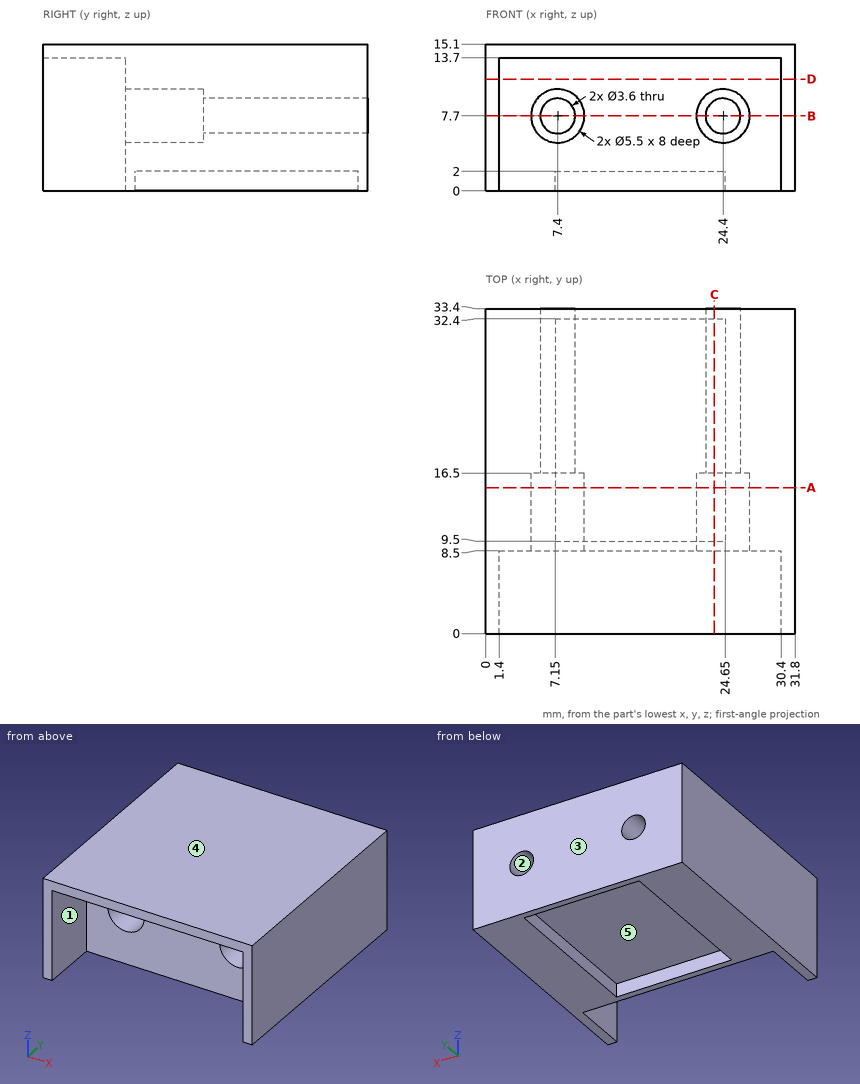
Geometry check sheet. Reference: drawing and pictorial views, mm from the part's lowest x, y, z. A direction names the side the tool comes from. Coordinates: 2 decimals unless noted, no trailing zeros. Order: outer loops, then holes, each group sorted by start corner. A loop starts at its lowest first (then second) coordinate and runs counter-clockwise, first axis right, second up. Notation, with made-up numbers: (41, -19.5) -> (78, -19.5) arc R19 ccw to (78, 2.5) -> close; hole circle Ø10 at (45, -16). An arc over 180 degrees is marked (long way). Use CSV: the item, a comma, the result in double quotes. Start each with the question number.
Q1. Section check C-C, the plane x = 23.5. Record the cut outline in (y, z), and give its area (3 significant figures).
Q2. Section check B-B, the plane z = 7.7. Record the cut outline in (x, y), and give its area (3 significant figures).
Q3. Section check D-D, the plane z = 11.5. Record the cut outline in (x, y), and give its area (3 significant figures).
Q4. Draft check along Y on the marked faces 3, 4 and 5. Enter one of: +Y half, -Y half, draft (parallel to the pull), parting line (faces both ways), or undercut.
Q5. Section check A-A, the plane y = 15. Record the cut outline in (x, z).
Q6. Thickness scan on line 1 along Z through (x, y) = (24.4, 11); line 2 along X through (y, z) = (4.5, 3.75); line 3 along Z through (x, y) = (24.4, 27.5). Record the ranges inside material, lowest first.
Q7. Depth check by flat-ended pin: P1, Ø4.5, axis at x = 23.5, z = 8, coming from the -Y side; P2, Ø4.5, axis at x = 7.4, z = 7.7, coming from the -Y side; P3, Ø2, axis at x = 24.4, z = 7.7, coming from the -Y side; P4, Ø5, axis at x = 13.5, y = 17.5, coming from the -Z side. Enter the tip coordinate at first touch or a pass-through.
Q8. Tool access check on the marked faces 1 and 2. Record the directions out of +Z, -Z, +X, -X, +Y, -Y that give a thin tool (end or side, any length) a straight path to the whole face; none if there is none.
Returned:
1,outline,"(0, 13.7) -> (8.5, 13.7) -> (8.5, 10.3) -> (16.5, 10.3) -> (16.5, 9.26) -> (33.4, 9.26) -> (33.4, 15.1) -> (0, 15.1) -> close; (8.5, 0) -> (9.5, 0) -> (9.5, 2) -> (32.4, 2) -> (32.4, 0) -> (33.4, 0) -> (33.4, 6.14) -> (16.5, 6.14) -> (16.5, 5.1) -> (8.5, 5.1) -> close"
1,area,"248 mm^2"
2,outline,"(0, 0) -> (1.4, 0) -> (1.4, 8.5) -> (4.65, 8.5) -> (4.65, 16.5) -> (5.6, 16.5) -> (5.6, 33.4) -> (0, 33.4) -> close; (9.2, 16.5) -> (10.15, 16.5) -> (10.15, 8.5) -> (21.65, 8.5) -> (21.65, 16.5) -> (22.6, 16.5) -> (22.6, 33.4) -> (9.2, 33.4) -> close; (26.2, 16.5) -> (27.15, 16.5) -> (27.15, 8.5) -> (30.4, 8.5) -> (30.4, 0) -> (31.8, 0) -> (31.8, 33.4) -> (26.2, 33.4) -> close"
2,area,"606 mm^2"
3,outline,"(0, 0) -> (1.4, 0) -> (1.4, 8.5) -> (30.4, 8.5) -> (30.4, 0) -> (31.8, 0) -> (31.8, 33.4) -> (0, 33.4) -> close"
3,area,"816 mm^2"
4,face 3,"+Y half"
4,face 4,"draft"
4,face 5,"undercut"
5,outline,"(0, 0) -> (7.15, 0) -> (7.15, 2) -> (24.65, 2) -> (24.65, 0) -> (31.8, 0) -> (31.8, 15.1) -> (0, 15.1) -> close; hole circle Ø5.5 at (7.4, 7.7); hole circle Ø5.5 at (24.4, 7.7)"
6,line 1,"z = 2 to 4.95, 10.45 to 15.1"
6,line 2,"x = 0 to 1.4, 30.4 to 31.8"
6,line 3,"z = 2 to 5.9, 9.5 to 15.1"
7,P1,"stops at y = 8.5"
7,P2,"stops at y = 16.5"
7,P3,"passes through"
7,P4,"stops at z = 2"
8,face 1,"-Z, -Y"
8,face 2,"+Y, -Y"
